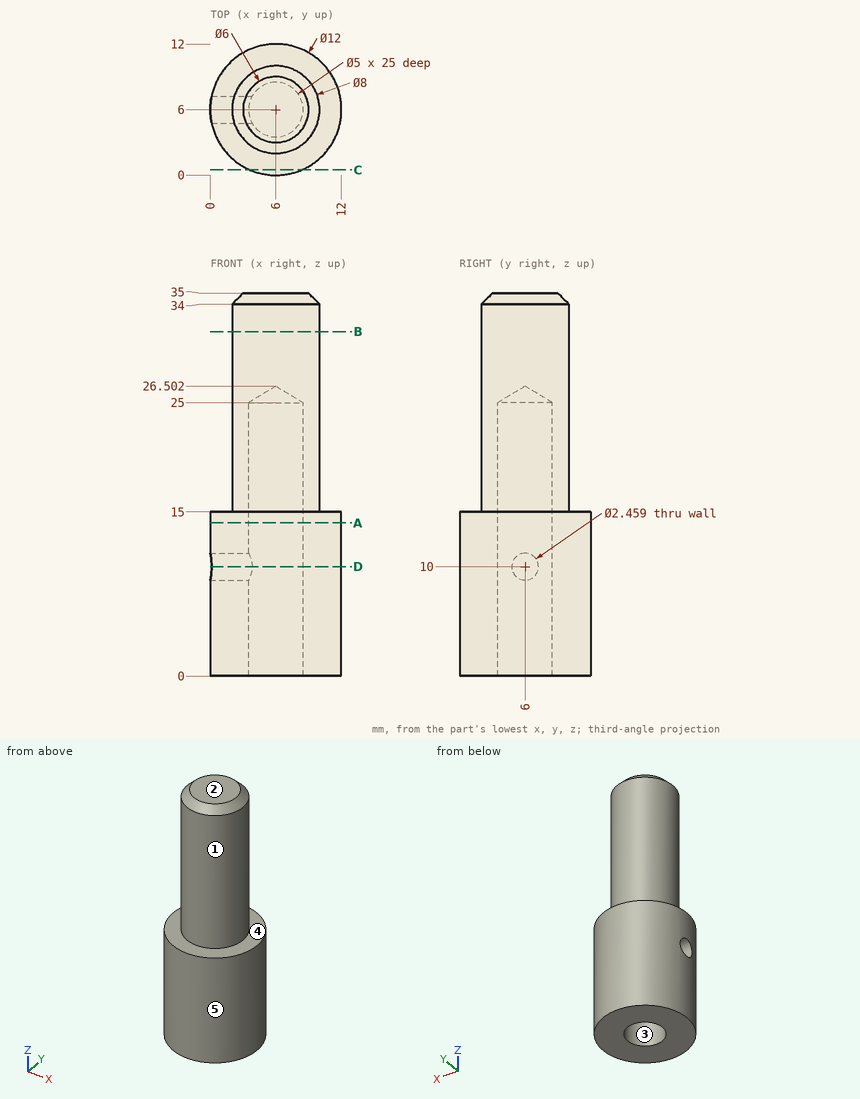
Could you check a few things on this drawing? It's one solid part, dimensions in mm from its lowest x, y, z. A direction names the side the tool comes from. Round coordinates to 2 decimals unless told otherwise and drop trailing zeros. Order: outer loops, then holes, each group sorted by start corner. A loop starts at its lowest first (then second) coordinate and runs counter-clockwise, first axis right, second up.
Q1. Imagine slicing it at B-B, the plane z = 31.5. List the corners of the cut face in (x, y) for me.
Geometry says:
outline: circle Ø8 at (6, 6)
Q2. Which directions (+Z, -Z, +X, -X, +Y, -Y) give clear straight access to the entire face, cutting with the end or side of a thin tool? Please do the marked faces 1 and 2.
Geometry says:
face 1: +Z
face 2: +Z, +X, -X, +Y, -Y
Q3. Please list where these lines run through material, in increasing order: probe 1 along Z at (x, y) = (9, 11); probe 2 along Y at (x, z) = (2.1, 10); probe 3 along X at (y, z) = (6.75, 13.5) (1 decimal).
Geometry says:
probe 1: z = 0 to 15
probe 2: y = 1.44 to 4.77, 7.23 to 10.56
probe 3: x = 0 to 3.6, 8.4 to 12
Q4. Imagine slicing it at A-A, the plane z = 14. List the corners of the cut face in (x, y) for me.
Geometry says:
outline: circle Ø12 at (6, 6); hole circle Ø5 at (6, 6)
Q5. I'm going to push flat-ended pins straight in: P1, Ø1.5, axis at x = 2, z = 23.5, coming from the -Y side; P2, Ø6, axis at y = 10, z = 15.5, coming from the -X side; P3, Ø6, axis at y = 10.5, z = 19, coming from the -X side. Where does each tip first touch, or does it pass through?
Geometry says:
P1: stops at y = 3.67
P2: stops at x = 0.09
P3: stops at x = 2.29
Q6. Imagine slicing it at D-D, the plane z = 10. List the corners of the cut face in (x, y) for me, then the cut area to 3 significant figures.
Geometry says:
outline: (0.13, 4.77) arc R6 ccw (long way) to (0.13, 7.23) - (3.82, 7.23) arc R2.5 cw (long way) to (3.82, 4.77) - close
area: 84.7 mm2
Q7. Imagine slicing it at C-C, the plane y = 0.5. List the corners of the cut face in (x, z) for me.
Geometry says:
outline: (3.6, 0) - (8.4, 0) - (8.4, 15) - (3.6, 15) - close
Q8. Thinking about a two-plate mould opening in Y: for the marked faces 3, 4 and 5, which applies, released by +Y, released by -Y, zero draft, split by the parting line, or undercut?
Geometry says:
face 3: undercut
face 4: zero draft
face 5: split by the parting line
